```python
from build123d import *

# Parameters (mm, degrees)
F0_W     = 1
F0_H     = 5
F1_DEPTH = 10
F2_R     = 0.49999


# Not quite as in the source:
# - a fillet or chamfer is up to 0.001 mm smaller than in the source, because OpenCascade refuses the exact size


with BuildPart() as f1:
    # F0 (on Right) → F1 (new body)
    with BuildSketch(Plane.YZ):
        Polygon((20, -5), (20, 10), (0, 10), (0, 0), (0, -5), align=None)
        with Locations((-0.5, -2.5)):
            Rectangle(F0_W, F0_H)
        with BuildLine():
            Line((-1, -5), (-1, 0))
            Line((-1, 0), (-1, 10))
            Line((-1, 10), (-11, 10))
            Line((-11, 10), (-11, 0))
            ThreePointArc((-11, 0), (-9.5355339059, -3.5355339059), (-6, -5))
            Line((-6, -5), (-1, -5))
        make_face()
    extrude(amount=F1_DEPTH)

    # F2 (radius 0.5 in the source; OpenCascade refuses exactly that, so slightly less here)
    f2_edges = [f1.edges().sort_by_distance(p)[0] for p in [
        (5, 0, 0),
        (5, -1, 0),
    ]]
    fillet(f2_edges, radius=F2_R)


solid = f1.part
```
Geometry check sheet. Reference: the model listing, model coordinates, mm. A direction names the side the tool comes from. Coordinates: 2 decimals unless noted, no trailing zeros. Write each loop counter-clockwise with the first axis right and the second up, starting at its lowest first coordinate (ties: lowest second). Pieces come first, ordered by that corner, then holes. Notation, with made-up numbers: M 31.25,10.5 L 39.25,10.5 A18 cw 39.25,38.5 Z; hole C 61.25,53.25 d3. An arc over 180 degrees is marked long. Answer as a JSON object with one key per item and string values.
1. Draft check along Y on faces 3 (the flat face through (5, -11, 5)), 4 (the flat face through (5, -1, 5)), 5 (the flat face through (5, 10, 10)). Enter one of: released by +Y, released by -Y, zero draft, split by the parting line, or undercut.
Answers below:
{"face 3": "released by -Y", "face 4": "undercut", "face 5": "zero draft"}
2. Section check D-D, the plane z = -3.25. Enter the section's corners in (x, y).
Answers below:
{"outline": "M 0,-9.8 L 10,-9.8 L 10,20 L 0,20 Z"}
3. Section check A-A, the plane z = 4. Enter the section's corners in (x, y), plus the area to 3 significant figures.
Answers below:
{"outline": "M 0,-11 L 10,-11 L 10,-1 L 0,-1 Z; M 0,0 L 10,0 L 10,20 L 0,20 Z", "area": "300 mm²"}
4. Scan lines: L1, parallel to Y at x = 3.75, z = 5.75; L2, parallel to Y at x = 5.75, z = -3; L3, parallel to Y at x = 3.25, z = -0.75. Record each from-to range of solid material in increasing order.
Answers below:
{"L1": "y = -11 to -1, 0 to 20", "L2": "y = -10 to 20", "L3": "y = -10.94 to 20"}
5. Tool access check on faces 1 (the flat face through (5, 0, 5)), 2 (the flat face through (0, 4, 3)). Record the directions out of +Z, -Z, +X, -X, +Y, -Y that give a thin tool (end or side, any length) a straight path to the whole face; none if there is none.
Answers below:
{"face 1": "+Z, +X, -X", "face 2": "+Z, -Z, -X, +Y, -Y"}
6. Section check C-C, the plane y = -9. Enter the section's corners in (x, z), plus the area to 3 significant figures.
Answers below:
{"outline": "M 0,-4 L 10,-4 L 10,10 L 0,10 Z", "area": "140 mm²"}
